Can you work these out from the model? Positions are in its coordinate system, mm. A direction names the side the tool comes from. Coordinates: 2 decimals unless noted, no trailing zeros. Write each loop counter-clockwise with the first axis right and the second up, starting at its lowest first coordinate (ties: lowest second). Pieces come first, ordered by that corner, then holes.
```python
from build123d import *

# Parameters (mm, degrees)
SKETCH1_R           = 18.25
BOSS_EXTRUDE1_DEPTH = 20
SKETCH2_R           = 10
BOSS_EXTRUDE2_DEPTH = 1.6
SKETCH3_R           = 3
BOSS_EXTRUDE3_DEPTH = 17.4
SKETCH4_W           = 0.25
SKETCH4_H           = 5
CIRPATTERN1_COUNT   = 3


with BuildPart() as part:
    # Sketch1 → Boss-Extrude1 (new body)
    with BuildSketch(Plane(origin=(0, 0, 0), x_dir=(1, 0, 0), z_dir=(0, 1, 0))):
        with Locations(Location((0, 0, 0), (0, 0, 270))):
            Circle(SKETCH1_R)
    extrude(amount=BOSS_EXTRUDE1_DEPTH)

    # Sketch2 → Boss-Extrude2 (add)
    with BuildSketch(Plane(origin=(0, 20, 0), x_dir=(1, 0, 0), z_dir=(0, 1, 0))):
        with Locations(Location((0, 0, 0), (0, 0, 270))):
            Circle(SKETCH2_R)
    extrude(amount=BOSS_EXTRUDE2_DEPTH)

    # Sketch3 → Boss-Extrude3 (add)
    with BuildSketch(Plane(origin=(0, 21.6, 0), x_dir=(1, 0, 0), z_dir=(0, 1, 0))):
        with Locations(Location((0, 0, 0), (0, 0, 270))):
            Circle(SKETCH3_R)
    extrude(amount=BOSS_EXTRUDE3_DEPTH)

    # Sketch4 → Cut-Revolve1 (revolve, cut)
    with BuildSketch(Plane(origin=(0, 0, 0), x_dir=(0, 0, -1), z_dir=(1, 0, 0)), mode=Mode.PRIVATE) as cut_revolve1_sk:
        with Locations((2.875, 29)):
            Rectangle(SKETCH4_W, SKETCH4_H)
    revolve(cut_revolve1_sk.sketch.rotate(Axis((0, 39, 0), (0, -1, 0)), 180), axis=Axis((0, 39, 0), (0, -1, 0)), mode=Mode.SUBTRACT)

    # Sketch7 → Ø3.0mm Dowel Hole1 (revolve, cut)
    with BuildSketch(Plane(origin=(0, 20, -15), x_dir=(0, 0, 1), z_dir=(1, 0, 0))):
        Polygon((0, 0), (0, 6.901290929), (1.5, 6), (1.5, 0), align=None)
    f_3_0mm_dowel_hole1 = revolve(axis=Axis((0, 26.35, -15), (0, -1, 0)), mode=Mode.SUBTRACT)

    # CirPattern1: Ø3.0mm Dowel Hole1 ×3 about axis
    cirpattern1_axis = Axis((0, 0, 0), (0, 1, 0))
    for i in range(1, CIRPATTERN1_COUNT):
        add(f_3_0mm_dowel_hole1.rotate(cirpattern1_axis, i * 360 / CIRPATTERN1_COUNT), mode=Mode.SUBTRACT)


solid = part.part
```
1. If we section it at A-A, the plane z = 0: List the corners of the cut face in (x, y) for me, plus the area to 3 significant figures.
2. Which directions (+Z, -Z, +X, -X, +Y, -Y) give clear straight access to the entire face, cutting with the end or side of a thin tool? Please do faces 4 (the face through (0.9, 35.2, 2.86)), 5 (the face through (-17.816, 9.86, -3.956)).
3. If I drill on L1, parallel to X at y = 16, z = 7; L2, parallel to X at y = 16.65, z = 7.5; L3, parallel to Y at x = -14.5, z = 9, over which ranges is the centre line in solid material (lowest first)?
4. I'm going to push flat-ended pins straight in: P1, Ø3, axis at y = 27, z = 6, coming from the -X side; P2, Ø10, axis at x = -7, z = 12, coming from the +Y side; P3, Ø2, axis at y = 5.5, z = -8, coming from the -X side; P4, Ø10, axis at y = 13, z = -5.5, coming from the +X side. Where does each tip first touch, or does it pass through?
5. If we section it at C-C, the plane x = -5.5: List the corners of the cut face in (y, z) for me, plus the area to 3 significant figures.
6. If we section it at B-B, the plane y = 35.5: List the corners of the cut face in (x, z) for me.
7. We'd pull the mould along Y, two halves only. Please class faces 1 (the face through (-8, 20, 8)), 2 (the face through (-0.07, 17.04, -16.5)), 3 (the face through (2.685, 29.035, -0.596)): released by +Y, released by -Y, zero draft, split by the parting line, or undercut.
8. If we section it at D-D, the plane y = 19: List the corners of the cut face in (x, z) for me, plus the area to 3 significant figures.
Answers:
1. outline: (-18.25, 0) - (18.25, 0) - (18.25, 20) - (10, 20) - (10, 21.6) - (3, 21.6) - (3, 26.5) - (2.75, 26.5) - (2.75, 31.5) - (3, 31.5) - (3, 39) - (-3, 39) - (-3, 31.5) - (-2.75, 31.5) - (-2.75, 26.5) - (-3, 26.5) - (-3, 21.6) - (-10, 21.6) - (-10, 20) - (-18.25, 20) - close
1. area: 864 mm2
2. face 4: +Y
2. face 5: +Y, -Y
3. L1: x = -16.85 to -14.4, -11.58 to 11.58, 14.4 to 16.85
3. L2: x = -16.64 to -14.49, -11.49 to 11.49, 14.49 to 16.64
3. L3: y = 0 to 20
4. P1: passes through
4. P2: stops at y = 21.6
4. P3: stops at x = -16.85
4. P4: stops at x = 18.24
5. outline: (0, -17.4) - (20, -17.4) - (20, -8.35) - (21.6, -8.35) - (21.6, 8.35) - (20, 8.35) - (20, 17.4) - (0, 17.4) - close
5. area: 723 mm2
6. outline: circle Ø6 at (0, 0)
7. face 1: released by +Y
7. face 2: zero draft
7. face 3: undercut
8. outline: circle Ø36.5 at (0, 0); hole circle Ø3 at (-12.99, 7.5); hole circle Ø3 at (0, -15); hole circle Ø3 at (12.99, 7.5)
8. area: 1,030 mm2
